Could you check a few things on this model? Use its own coordinates, in mm. Face numbers are marked on the shaded views. A direction names the side the tool comes from. Round coordinates to 2 decimals unless told otherwise and drop trailing zeros. Write each loop counter-clockwise with the first axis right and the second up, starting at its lowest first coordinate (ties: lowest second). Pieces come first, ordered by that corner, then holes. Notation, with made-up numbers: (60.5, -0.5) - (100.5, -0.5) arc R19 ccw to (100.5, 17.5) - close; hole circle Ø4 at (70.5, -20). An arc over 180 degrees is marked (long way). Write each question's results on one line, items separated by ' | '. Start each with the question number.
(1) Please list where these lines run through material, in increasing order: line 1 (Z direction, x = 7.25, y = -6); line 2 (Y direction, x = 0.5, z = -1.5); line 3 (Y direction, x = 3, z = 0.25). Write a range as [from, to].
(2) On a 3-axis mill with a long thin cutter (end or side, diameter ignored), from which of +Z, -Z, +X, -X, +Y, -Y can I reach the whole of each face in a straight line? I mean the marked faces 1, 2, 3 and 4. Say none if no direction works.
(3) Imagine slicing it at D-D on y = 6.5. Write out the boundary of the cut face in (x, z).
(4) Thinking about a two-plate mould opening in Y: for the marked faces 5, 6, 7 and 8, which applies, +Y half, -Y half, draft (parallel to the pull), parting line (faces both ways), or undercut?
(5) For P1, Ø4, axis at y = 11.69, z = -1.55, coming from the +X side; P2, Ø4.5, axis at x = 2.5, z = -7.5, coming from the -Y side; P3, Ø1.6, axis at x = 4.5, z = 4, coming from the -Y side; P4, Ø4, axis at x = 7, z = -8.5, coming from the -Y side, each with a flat end and sliding along its axis, tell me the tip position at first contact or that it passes through.
(6) Imagine slicing it at A-A on z = 6. Write out the boundary of the cut face in (x, y).
(7) Imagine slicing it at C-C on y = 9.5. Write out the boundary of the cut face in (x, z), then the cut area to 3 significant figures.
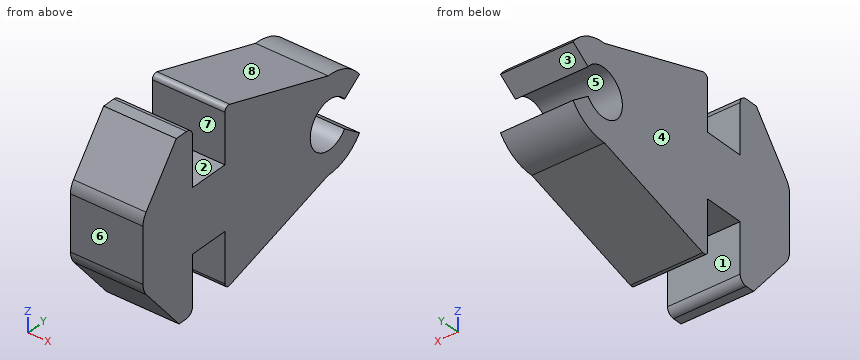
```python
from build123d import *

# Parameters (mm, degrees)
F0_R     = 2.55
F1_DEPTH = 7.8
F2_R     = 0.5
F4_DEPTH = 25


with BuildPart() as f1:
    # F0 (on Right) → F1 (new body)
    with BuildSketch(Plane.YZ):
        with BuildLine():
            Line((-2.326186, 7.823175), (-2.326186, 1.823175))
            Line((-2.326186, 1.823175), (-6.690186, 1.823175))
            Line((-6.690186, 1.823175), (-6.690186, 7.146175))
            ThreePointArc((-6.690186, 7.146175), (-6.9245, 7.71186), (-7.490186, 7.946175))
            Line((-7.490186, 7.946175), (-8.86261, 7.946175))
            Line((-8.86261, 7.946175), (-12.92499, 2.634016))
            ThreePointArc((-12.92499, 2.634016), (-13.23068, 2.06042), (-13.336295, 1.419089))
            Line((-13.336295, 1.419089), (-13.336295, -4.483028))
            ThreePointArc((-13.336295, -4.483028), (-13.217831, -5.161131), (-12.876472, -5.758903))
            Line((-12.876472, -5.758903), (-8.490186, -11.053825))
            Line((-8.490186, -11.053825), (-7.490186, -11.053825))
            ThreePointArc((-7.490186, -11.053825), (-6.9245, -10.819511), (-6.690186, -10.253825))
            Line((-6.690186, -10.253825), (-6.690186, -4.930825))
            Line((-6.690186, -4.930825), (-2.326186, -4.930825))
            Line((-2.326186, -4.930825), (-2.326186, -10.930825))
            Line((-2.326186, -10.930825), (11.55518, -6.601922))
            ThreePointArc((11.55518, -6.601922), (16.743814, -1.552504), (11.552539, 3.494198))
            Line((11.552539, 3.494198), (-2.326186, 7.823175))
        make_face()
        with Locations((11.693814, -1.553825)):
            Circle(F0_R, mode=Mode.SUBTRACT)
    extrude(amount=F1_DEPTH)

    # F2
    f2_edges = [f1.edges().sort_by_distance(p)[0] for p in [
        (3.9, -2.326186, 7.823175),
        (3.9, -2.326186, -10.930825),
    ]]
    fillet(f2_edges, radius=F2_R)

    # F3 (on face) → F4 (cut)
    with BuildSketch(Plane.YZ.offset(7.8)):
        Polygon((19.312905, 3.981768), (11.693814, -1.553825), (19.312905, -7.089419), align=None)
    extrude(amount=-F4_DEPTH, mode=Mode.SUBTRACT)


solid = f1.part
```
Response:
1) line 1: [-4.93, 1.82] | line 2: [-13.34, 9.14] | line 3: [-13.34, 9.89], [13.5, 14.18]
2) face 1: -Z, +X, -X | face 2: +Z, +X, -X | face 3: +X, -X, +Y | face 4: +Z, -Z, -X, +Y, -Y
3) outline: (0, -8.18) - (7.8, -8.18) - (7.8, 5.07) - (0, 5.07) - close
4) face 5: undercut | face 6: -Y half | face 7: undercut | face 8: +Y half
5) P1: through | P2: y = -13.18 | P3: y = -12.49 | P4: y = -12.26
6) outline: (0, -10.35) - (7.8, -10.35) - (7.8, -6.69) - (0, -6.69) - close; (0, -2.33) - (7.8, -2.33) - (7.8, 3.52) - (0, 3.52) - close
7) outline: (0, -7.24) - (7.8, -7.24) - (7.8, -2.85) - (0, -2.85) - close; (0, -0.25) - (7.8, -0.25) - (7.8, 4.13) - (0, 4.13) - close | area: 68.5 mm²
